Geometry check sheet. Reference: the model listing, model coordinates, mm. Face numbers are marked on the shaded views. A direction names the side the tool comes from. Coordinates: 2 decimals unless noted, no trailing zeros. Write each loop counter-clockwise with the first axis right and the second up, starting at its lowest first coordinate (ties: lowest second). Pieces come first, ordered by that corner, then holes.
from build123d import *

# Parameters (mm, degrees)
F0_R      = 14
F1_DEPTH  = 3.4
F3_R      = 12.5
F4_DEPTH  = 50
F6_R      = 8.05
F7_DEPTH  = 40
F9_R      = 6.25
F10_DEPTH = 66.1


# Not quite as in the source:
# - a fillet or chamfer that OpenCascade refuses, or shapes differently, is made with other operations: its cross-section is extruded or revolved along the edge and cut away or added


with BuildPart() as f1:
    # F0 (on Front) → F1 (new body)
    with BuildSketch(Plane.XZ):
        Circle(F0_R)
    extrude(amount=F1_DEPTH)

    # F3 (on offset) → F4 (join)
    with BuildSketch(Plane.XZ.offset(3.4)):
        Circle(F3_R)
    extrude(amount=F4_DEPTH)

    # F6 (on offset) → F7 (cut)
    with BuildSketch(Plane.XZ.offset(53.4)):
        Circle(F6_R)
    extrude(amount=-F7_DEPTH, mode=Mode.SUBTRACT)

    # F8: chamfer of 5 on 1 edges, made by hand

    # F8_s1 → F8_t2 (revolve, cut)
    with BuildSketch(Plane.XY):
        Polygon((12.5, -48.4), (7.5, -53.4), (12.5, -53.4), align=None)
    revolve(axis=Axis((0, -53.4, 0), (0, -1, 0)), mode=Mode.SUBTRACT)

    # F9 (on Front) → F10 (cut)
    with BuildSketch(Plane.XZ):
        Circle(F9_R)
    extrude(amount=F10_DEPTH, mode=Mode.SUBTRACT)


solid = f1.part
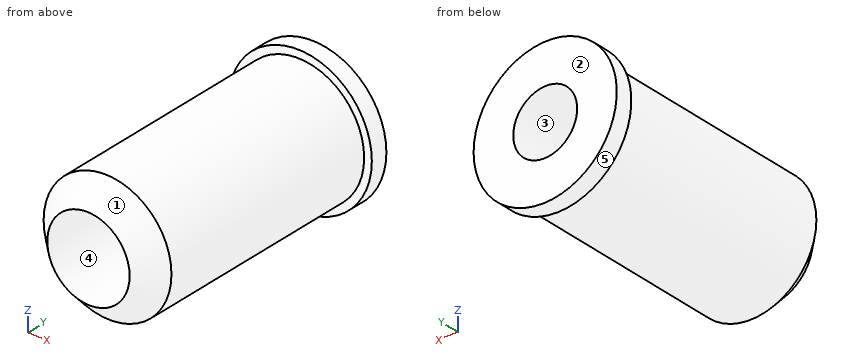
1. Sectioned sample at A-A, the plane x = 0. Record the boundary of the cut face in (y, z), and give its area (3 significant figures).
Computed values:
outline: (-52.85, -8.05) - (-48.4, -12.5) - (-3.4, -12.5) - (-3.4, -14) - (0, -14) - (0, -6.25) - (-13.4, -6.25) - (-13.4, -8.05) - close; (-52.85, 8.05) - (-13.4, 8.05) - (-13.4, 6.25) - (0, 6.25) - (0, 14) - (-3.4, 14) - (-3.4, 12.5) - (-48.4, 12.5) - close
area: 509 mm2
2. Draft check along X on the marked faces 1, 2 and 3. Enter one of: released by +X, released by -X, zero draft, split by the parting line, or undercut.
Computed values:
face 1: split by the parting line
face 2: zero draft
face 3: undercut
3. Access from +Z, -Z, +X, -X, +Y, -Y to the whole of each face (thin tool, end or side, straight path). Record for the marked faces 4 and 5.
Computed values:
face 4: -Y
face 5: +Y, -Y
4. Thickness scan on line 1 along Z through (x, y) = (0, -7.5); line 2 along Z through (x, y) = (0, -3); line 3 along Y through (x, z) = (6.75, 3.25). Record the ranges inside material, lowest first.
Computed values:
line 1: z = -12.5 to -6.25, 6.25 to 12.5
line 2: z = -14 to -6.25, 6.25 to 14
line 3: y = -13.4 to 0
5. Sectioned sample at B-B, the plane z = 0. Record the boundary of the cut face in (x, y), and give its area (3 significant figures).
Computed values:
outline: (-14, -3.4) - (-12.5, -3.4) - (-12.5, -48.4) - (-8.05, -52.85) - (-8.05, -13.4) - (-6.25, -13.4) - (-6.25, 0) - (-14, 0) - close; (6.25, -13.4) - (8.05, -13.4) - (8.05, -52.85) - (12.5, -48.4) - (12.5, -3.4) - (14, -3.4) - (14, 0) - (6.25, 0) - close
area: 509 mm2
6. Sectioned sample at C-C, the plane y = -28. Record the boundary of the cut face in (x, z).
Computed values:
outline: circle Ø25 at (0, 0); hole circle Ø16.1 at (0, 0)
7. Gauge pin test, flat ends, axial feed: pin 1 Ø5 at (y, z) = (-22, 0.5) entering from +X; pin 2 Ø6 at (x, y) = (-2.5, -10.5) entering from -Z; pin 3 Ø3 at (y, z) = (-47, 3.5) entering from +X. Record the tip position at first contact, or that the pin passes through.
Computed values:
pin 1: stops at x = 12.5
pin 2: stops at z = -12.5
pin 3: stops at x = 12.34
